Verification items for this drawing (mm, ordinates from the low corner). Round coordinates to 2 decimals unless told otherwise and drop trailing zeros. Order: outer loops, then holes, each group sorted by start corner. A loop starts at its lowest first (then second) coordinate and runs counter-clockwise, first axis right, second up. Notation, with made-up numbers: M 57.25,74 L 75.25,74 A21 ccw 75.25,88 Z; hole C 63,-3 d11. An arc over 180 degrees is marked long. Return JSON: item names as keys, results as strings. Group by question number.
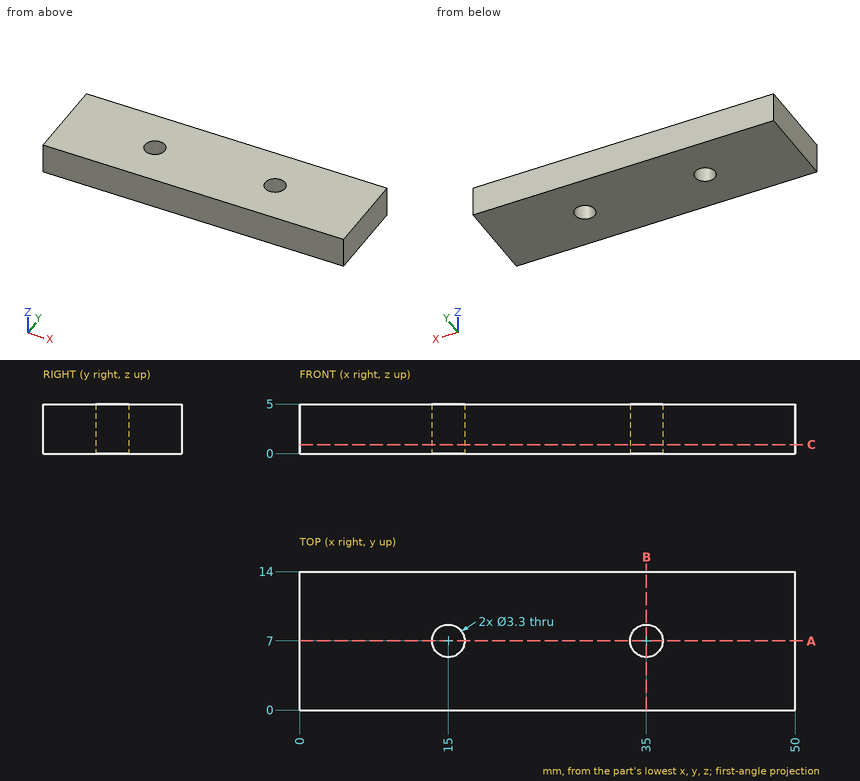
1. Thickness scan on line 1 along Y through (x, z) = (35, 3.7); line 2 along X through (y, z) = (8.5, 3.85); line 3 along X through (y, z) = (7.25, 3.8). Record the ranges inside material, lowest first. Write a range as from..to.
2. Cross-section at C-C (z = 0.9). Enter the section's corners in (x, y).
3. Cross-section at B-B (x = 35). Enter the section's corners in (y, z).
4. Go/stop test with a flat-tipped pin: pin 1 (3 mm diameter, centred on x = 15, y = 7, fed in from -Z). Record where the tip stops, or that it passes through.
5. Cross-section at A-A (y = 7). Enter the section's corners in (x, z), plus the area to 3 significant figures.
Computed:
{
 "1": {"line 1": "y = 0..5.35, 8.65..14", "line 2": "x = 0..14.31, 15.69..34.31, 35.69..50", "line 3": "x = 0..13.37, 16.63..33.37, 36.63..50"},
 "2": {"outline": "M 0,0 L 50,0 L 50,14 L 0,14 Z; hole C 15,7 d3.3; hole C 35,7 d3.3"},
 "3": {"outline": "M 0,0 L 5.35,0 L 5.35,5 L 0,5 Z; M 8.65,0 L 14,0 L 14,5 L 8.65,5 Z"},
 "4": {"pin 1": "passes through"},
 "5": {"outline": "M 0,0 L 13.35,0 L 13.35,5 L 0,5 Z; M 16.65,0 L 33.35,0 L 33.35,5 L 16.65,5 Z; M 36.65,0 L 50,0 L 50,5 L 36.65,5 Z", "area": "217 mm²"}
}
